Source: CAD feature listing. Evaluate the final solid. Frame: model axes, mm. Face numbers are marked on the shaded views. A direction names the side the tool comes from. Coordinates: 2 decimals unless noted, no trailing zeros. Loops run counter-clockwise (first coordinate to the right, second up) from the corner with the lowest first, then second, coordinate; pieces in that order, holes last.
Item 1: Section query B-B, the plane x = 14. Return the cut outline in (y, z), then the cut area to 3 significant figures.
Item 2: Section query A-A, the plane y = 12. Return the cut outline in (x, z).
Item 3: Line query: probe 1 along X at (y, z) = (6, -32); probe 2 along X at (y, z) = (28, -29); probe 3 along Y at (x, z) = (87, -7.5). Output: solid intervals per line, ascending.
Item 4: Section query C-C, the plane z = 22. Return the cut outline in (x, y).
Item 5: Pull-direction query (Y, two-part tool) for the marked faces 1, 2 and 3; classes: +Y half, -Y half, draft (parallel to the pull), parting line (faces both ways), or undercut.
Item 6: Reachability of the marked faces 4, 5 and 6 from +Z, -Z, +X, -X, +Y, -Y: full face, straight path, thin tool, end or side. Return the list, or none.
Item 7: Section query D-D, the plane y = 24. Return the cut outline in (x, z).
Item 8: Pin query (flat end, axial travel): pin 1 Ø2 at (y, z) = (3, 0) entering from -X; pin 2 Ø9.5 at (x, z) = (20, 27) entering from +Y; pin 3 Ø3 at (y, z) = (7, -1) entering from -X; pin 4 Ø1 at (y, z) = (7.5, 3) entering from +X. Return the tip coordinate at first contact, or that it passes through.
```python
from build123d import *

# Parameters (mm, degrees)
SKETCH1_W           = 95
SKETCH1_H           = 75
BOSS_EXTRUDE1_DEPTH = 100
CUT_EXTRUDE1_DEPTH  = 40
SKETCH4_W           = 35
SKETCH4_H           = 35
CUT_EXTRUDE2_DEPTH  = 96
BOSS_EXTRUDE4_DEPTH = 6


with BuildPart() as part:
    # Sketch1 → Boss-Extrude1 (new body)
    with BuildSketch(Plane(origin=(0, 0, 0), x_dir=(0, 0, -1), z_dir=(1, 0, 0))):
        Rectangle(SKETCH1_W, SKETCH1_H)
    extrude(amount=BOSS_EXTRUDE1_DEPTH)

    # Sketch2 → Cut-Extrude1 (cut)
    with BuildSketch(Plane(origin=(100, 0, 0), x_dir=(0, 0, -1), z_dir=(1, 0, 0))):
        with BuildLine():
            Line((37.5, 37.5), (11.116502976, 7.057503434))
            ThreePointArc((11.116502976, 7.057503434), (-3.835336242, 2.323958076), (-6.395690793, -13.148873992))
            Line((-6.395690793, -13.148873992), (-27.5, -37.5))
            Line((-27.5, -37.5), (-47.5, -37.5))
            Line((-47.5, -37.5), (-47.5, 37.5))
            Line((-47.5, 37.5), (37.5, 37.5))
        make_face()
    extrude(amount=-CUT_EXTRUDE1_DEPTH, mode=Mode.SUBTRACT)

    # Sketch4 → Cut-Extrude2 (cut, through all)
    with BuildSketch(Plane.XY.offset(47.5)):
        with Locations((17.5, 20)):
            Rectangle(SKETCH4_W, SKETCH4_H)
    extrude(amount=-CUT_EXTRUDE2_DEPTH, mode=Mode.SUBTRACT)

    # Sketch14 → Boss-Extrude4 (add)
    with BuildSketch(Plane.XY.offset(9.5)):
        Polygon((35, 37.5), (0, 2.5), (35, 2.5), align=None)
    extrude(amount=BOSS_EXTRUDE4_DEPTH)


solid = part.part
```
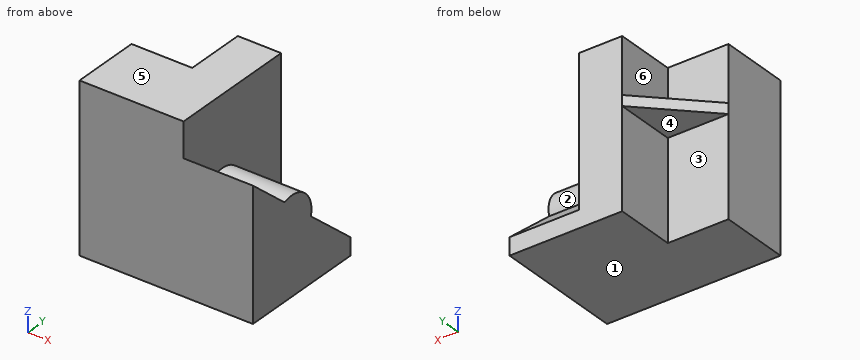
Verdict:
1. outline: (-37.5, -47.5) - (2.5, -47.5) - (2.5, 9.5) - (16.5, 9.5) - (16.5, 15.5) - (2.5, 15.5) - (2.5, 47.5) - (-37.5, 47.5) - close
1. area: 3,880 mm2
2. outline: (9.5, 9.5) - (35, 9.5) - (35, -47.5) - (100, -47.5) - (100, -15.4) - (60, -15.4) - (60, 47.5) - (35, 47.5) - (35, 15.5) - (9.5, 15.5) - close
3. probe 1: x = 35 to 100
3. probe 2: x = 35 to 60
3. probe 3: y = -37.5 to 7.5
4. outline: (0, -37.5) - (100, -37.5) - (100, -31.15) - (60, -31.15) - (60, 37.5) - (35, 37.5) - (35, 2.5) - (0, 2.5) - close
5. face 1: draft
5. face 2: undercut
5. face 3: +Y half
6. face 4: -Z, -X, +Y
6. face 5: +Z, +X, -X, +Y, -Y
6. face 6: +Z, -X, +Y
7. outline: (21.5, 9.5) - (35, 9.5) - (35, -47.5) - (100, -47.5) - (100, -25.8) - (60, -25.8) - (60, 47.5) - (35, 47.5) - (35, 15.5) - (21.5, 15.5) - close
8. pin 1: stops at x = 0
8. pin 2: stops at y = 2.5
8. pin 3: stops at x = 35
8. pin 4: stops at x = 60
